Read the model definition and answer for the solid it produces. Units are mm, in the model's axes. A direction names the side the tool comes from. Round coordinates to 2 decimals unless told otherwise and drop trailing zeros. Loops run counter-clockwise (first coordinate to the right, second up) from the corner with the lowest first, then second, coordinate; pieces in that order, holes last. Notation, with made-up numbers: (1.5, -12.75) - (7.5, -12.75) arc R12 ccw to (7.5, -5.75) - close; hole circle Ø10 at (2.5, -37). An arc over 180 degrees is marked (long way). Use CSV: the item, a comma, the result in double quotes. Start each with the question number.
1. Consider line 1 along Z through (x, y) = (125, 8); line 2 along Y through (x, z) = (75, 8.5); line 3 along X through (y, z) = (6, 20). Determine where each line is inside the solid, lowest interval first.
2. A tool of negligible diameter and unlimited length cuts with its end or side. For faces 1 (the flat face through (99, 42, 20)), 2 (the cylindrical face through (147.353, 57.681, 10.14)), from which of +Z, -Z, +X, -X, +Y, -Y can it reach the whole face along a straight path? Write none if from no direction.
3. Find section A-A (x = 125). Give the vertices of the cut face in (y, z).
4. Find section D-D (z = 22). Give the vertices of the cut face in (x, y), and give its area (3 significant figures).
5. Find section C-C (y = 56). Give the vertices of the cut face in (x, z).
6. Determine the mould class of faces 3 (the cylindrical face through (10.76, 9.86, 23.46)), 4 (the flat face through (91, 28, 0)), 5 (the flat face through (50, 35, 10)) for opening direction X: +X half, -X half, draft (parallel to the pull), parting line (faces both ways), or undercut.
7. Find section B-B (z = 7.5). Give the vertices of the cut face in (x, y), and give its area (3 significant figures).
8. Given pin 1 Ø6 at (y, z) = (31, 6.5) entering from -X; pin 2 Ø4 at (y, z) = (9, 23) entering from -X; pin 3 Ø18 at (x, z) = (20, 19.63) entering from +Y; pin 4 Ø3 at (x, y) = (76, 26.5) entering from +Z, each flat-ended and moving along its own axis, determine where each tip first touches the part or whether it passes through.
from build123d import *

# Parameters (mm, degrees)
EXTRUDE_1_DEPTH         = 20
EXTRUDE_2_DEPTH         = 20
FILLET_1_R              = 12
FILLET_2_R              = 20
FILLET_3_R              = 25
HOLE_WIZARD_20_0_20_1_D = 20
HOLE_WIZARD_20_0_20_2_D = 20


with BuildPart() as part:
    # 草圖1 → 填料-伸長1 (new body)
    with BuildSketch(Plane(origin=(0, 0, 0), x_dir=(1, 0, 0), z_dir=(0, 1, 0))):
        Polygon((0, 0), (150, 0), (150, -75), (0, -35), align=None)
    extrude(amount=EXTRUDE_1_DEPTH)

    # 草圖2 → 填料-伸長2 (add)
    with BuildSketch(Plane(origin=(0, 0, 0), x_dir=(-1, 0, 0), z_dir=(0, 0, -1))):
        Polygon((-150, 0), (-150, 60), (-50, 80), (-50, 0), align=None)
    extrude(amount=-EXTRUDE_2_DEPTH)

    # 圓角1
    fillet_1_edges = [part.edges().sort_by_distance(p)[0] for p in [
        (150, 60, 10),
    ]]
    fillet(fillet_1_edges, radius=FILLET_1_R)

    # 圓角2
    fillet_2_edges = [part.edges().sort_by_distance(p)[0] for p in [
        (0, 10, 35),
    ]]
    fillet(fillet_2_edges, radius=FILLET_2_R)

    # 圓角3
    fillet_3_edges = [part.edges().sort_by_distance(p)[0] for p in [
        (50, 80, 10),
        (150, 10, 75),
    ]]
    fillet(fillet_3_edges, radius=FILLET_3_R)

    # Ø20.0 (20) 直徑孔1 (through all)
    with Locations(Plane(origin=(0, 20, 0), x_dir=(1, 0, 0), z_dir=(0, 1, 0))):
        with Locations((125, -42.45970884), (20, -19.634433738)):
            Hole(HOLE_WIZARD_20_0_20_1_D / 2)

    # Ø20.0 (20) 直徑孔2 (through all)
    with Locations(Plane.XY.offset(20)):
        with Locations((75, 49.504902432)):
            Hole(HOLE_WIZARD_20_0_20_2_D / 2)


solid = part.part
Filled sheet:
1,line 1,"z = 0 to 32.46, 52.46 to 67.46"
1,line 2,"y = 0 to 39.5, 59.5 to 74.5"
1,line 3,"x = 0 to 10.01, 29.99 to 150"
2,face 1,"+Z, +X, -X, +Y"
2,face 2,"+Z, -Z, +X, +Y"
3,outline,"(0, 0) - (65, 0) - (65, 20) - (20, 20) - (20, 32.46) - (0, 32.46) - close; (0, 52.46) - (20, 52.46) - (20, 67.46) - (0, 67.46) - close"
4,outline,"(0.14, 0) - (10.28, 0) - (10.28, 20) - (0.14, 20) - close; (29.72, 0) - (150, 0) - (150, 20) - (29.72, 20) - close"
4,area,"2,610 mm²"
5,outline,"(50.86, 0) - (67.4, 0) - (67.4, 20) - (50.86, 20) - close; (82.6, 0) - (148.48, 0) - (148.48, 20) - (82.6, 20) - close"
6,face 3,"undercut"
6,face 4,"draft"
6,face 5,"-X half"
7,outline,"(0, 0) - (150, 0) - (150, 50.16) arc R12 ccw to (140.35, 61.93) - (79.9, 74.02) arc R25 ccw to (50, 49.5) - (50, 20) - (0, 20) - close; hole circle Ø20 at (75, 49.5)"
7,area,"7,460 mm²"
8,pin 1,"stops at x = 50"
8,pin 2,"stops at x = 0.05"
8,pin 3,"passes through"
8,pin 4,"stops at z = 20"
